Autodesk Inventor part; units mm, degrees
ref_plane "YZ Plane" through (0, 0, 0) normal (1, 0, 0) x (0, 1, 0)
ref_plane "XZ Plane" through (0, 0, 0) normal (0, 1, 0) x (-1, 0, 0)
ref_plane "XY Plane" through (0, 0, 0) normal (0, 0, 1) x (1, 0, 0)
sketch "Sketch1" plane through (0, 0, 0) normal (0, 1, 0) x (-1, 0, 0)
  line L0 (7.9003, 23.0254) -> (-242.0997, 23.0254)
  line L1 (-242.0997, 23.0254) -> (-242.0997, -336.9746)
  line L2 (-242.0997, -336.9746) -> (7.9003, -336.9746)
  line L3 (7.9003, -336.9746) -> (7.9003, 23.0254)
  point P0 (0, 0)
  dimension "d0" = 250
  dimension "d1" = 360
extrude "Extrusion1" add sketch "Sketch1" along normal blind 52
shell "Shell1" thickness 15 removed faces 1 at (158.7664, 52, -96.9746)
sketch3d "3D Sketch5"
properties part number "Part1proj" material "Wood (Birch)"
Model file for the job. Use its own axes, mm. A direction names the side the tool comes from. Give positions to 0.01 mm unless a question says otherwise; leave off trailing zeros. Loops run counter-clockwise (first coordinate to the right, second up) from the corner with the lowest first, then second, coordinate; pieces in that order, holes last.
Item 1: Drop flat-ended pins along their axis: P1, Ø3, axis at x = 52, z = -65.5, coming from the +Y side; P2, Ø8, axis at x = 214, z = -116, coming from the -Y side. Give the stop position or say it passes through.
Check values:
P1: stops at y = 15
P2: stops at y = 0
Item 2: Slice it at A-A (x = 50). Write the cut outline in (y, z), plus the area to 3 significant figures.
Check values:
outline: (0, -336.97) - (52, -336.97) - (52, -321.97) - (15, -321.97) - (15, 8.03) - (52, 8.03) - (52, 23.03) - (0, 23.03) - close
area: 6,510 mm2
Item 3: Which spindle directions (+Z, -Z, +X, -X, +Y, -Y) get a long thin tool onto all of the face, cutting with end or side? Do faces 1 (the face through (116, 33, 8.025)), 2 (the face through (242.1, 26, -154)). Say none if no direction does.
Check values:
face 1: +Y
face 2: +Z, -Z, +X, +Y, -Y
Item 4: Slice it at B-B (y = 42.5). Write the cut outline in (x, z), plus the area to 3 significant figures.
Check values:
outline: (-7.9, -336.97) - (242.1, -336.97) - (242.1, 23.03) - (-7.9, 23.03) - close; hole (7.1, -321.97) - (227.1, -321.97) - (227.1, 8.03) - (7.1, 8.03) - close
area: 17,400 mm2
Item 5: Mould opens along Z. For faces 3 (the face through (119, 26, -336.975)), 4 (the face through (119, 0, -154)), 5 (the face through (119, 33, -321.975)) say: +Z half, -Z half, draft (parallel to the pull), parting line (faces both ways), or undercut.
Check values:
face 3: -Z half
face 4: draft
face 5: undercut
Item 6: Slice it at C-C (z = -93). Write the cut outline in (x, y).
Check values:
outline: (-7.9, 0) - (242.1, 0) - (242.1, 52) - (227.1, 52) - (227.1, 15) - (7.1, 15) - (7.1, 52) - (-7.9, 52) - close
Item 7: Drill centre lines: line 1 along X through (y, z) = (28.5, -99.5); line 2 along Z through (x, y) = (22, 18.5); line 3 along Y through (x, z) = (199, -214.5). Where is each one in solid material? Low to high.
Check values:
line 1: x = -7.9 to 7.1, 227.1 to 242.1
line 2: z = -336.97 to -321.97, 8.03 to 23.03
line 3: y = 0 to 15
